```python
from build123d import *

# Parameters (mm, degrees)
BOSS_EXTRUDE1_DEPTH = 9
FILLET1_R           = 6
FILLET2_R           = 4
BOSS_EXTRUDE2_DEPTH = 18
LPATTERN1_COUNT     = 6
LPATTERN1_PITCH     = 6
CUT_EXTRUDE1_DEPTH  = 149.120803233
CUT_EXTRUDE2_DEPTH  = 8
SKETCH6_R           = 1.5
CUT_EXTRUDE3_DEPTH  = 149.120803233
SKETCH7_R           = 1.75
BOSS_EXTRUDE3_DEPTH = 3
SKETCH9_R           = 1.25
CUT_EXTRUDE4_DEPTH  = 1
SKETCH10_R          = 1.25
CUT_EXTRUDE5_DEPTH  = 1
CUT_EXTRUDE7_DEPTH  = 1


with BuildPart() as part:
    # Sketch2 → Boss-Extrude1 (new, symmetric)
    with BuildSketch(Plane(origin=(0, 0, 0), x_dir=(1, 0, 0), z_dir=(0, 1, 0))):
        with BuildLine():
            Line((-39.563995826, -83.832935468), (-42.630019208, -84.799815256))
            Line((-42.630019208, -84.799815256), (-45.240501853, -94.451735935))
            Line((-45.240501853, -94.451735935), (-34.884360154, -102.309873698))
            Line((-34.884360154, -102.309873698), (-25.888982114, -130.929502869))
            Line((-25.888982114, -130.929502869), (-25.888982114, -137.929502869))
            Line((-25.888982114, -137.929502869), (-14.888982114, -137.929502869))
            Line((-14.888982114, -137.929502869), (-14.888982114, -87.929502869))
            Line((-14.888982114, -87.929502869), (-6.735604792, -82.139646373))
            ThreePointArc((-6.735604792, -82.139646373), (-0.446003435, -73.378982845), (-11.226689216, -73.670744316))
            Line((-11.226689216, -73.670744316), (-21.363708344, -80.271037279))
            Line((-21.363708344, -80.271037279), (-28.269041415, -80.271037279))
            Line((-28.269041415, -80.271037279), (-28.269041415, -9.271037279))
            Line((-28.269041415, -9.271037279), (-51.831492155, -13.832935468))
            Line((-51.831492155, -13.832935468), (-39.563995826, -83.832935468))
        make_face()
    extrude(amount=BOSS_EXTRUDE1_DEPTH, both=True)

    # Fillet1
    fillet1_edges = [part.edges().sort_by_distance(p)[0] for p in [
        (-51.831492155, 0, 13.832935468),
        (-28.269041415, 0, 9.271037279),
    ]]
    fillet(fillet1_edges, radius=FILLET1_R)

    # Fillet2
    fillet2_edges = [part.edges().sort_by_distance(p)[0] for p in [
        (-42.630019208, 0, 84.799815256),
        (-25.888982114, 0, 137.929502869),
        (-45.240501853, 0, 94.451735935),
    ]]
    fillet(fillet2_edges, radius=FILLET2_R)

    # Sketch3 → Boss-Extrude2 (add)
    with BuildSketch(Plane(origin=(0, 9, 0), x_dir=(1, 0, 0), z_dir=(0, 1, 0))):
        Polygon((-14.888982114, -130.986597937), (-14.888982114, -134.986597937), (-10.884332588, -132.931354664), align=None)
    boss_extrude2 = extrude(amount=-BOSS_EXTRUDE2_DEPTH)

    # LPattern1: Boss-Extrude2 ×6
    with Locations(*[(0, 0, -i * LPATTERN1_PITCH) for i in range(1, LPATTERN1_COUNT)]):
        add(boss_extrude2)

    # Sketch4 → Cut-Extrude1 (cut, through all)
    with BuildSketch(Plane(origin=(0, 9, 0), x_dir=(1, 0, 0), z_dir=(0, 1, 0))):
        Polygon((-16.683079676, -131.183487283), (-16.683079676, -106.183487283), (-31.683079676, -106.183487283), align=None)
    extrude(amount=-CUT_EXTRUDE1_DEPTH, mode=Mode.SUBTRACT)

    # Sketch5 → Cut-Extrude2 (cut)
    with BuildSketch(Plane(origin=(-61.013660914, 0, 19.177080956), x_dir=(0.29984593468383275, 0, 0.9539876390465334), z_dir=(-0.9539876390465333, 0, 0.2998459346838327))):
        Polygon((94.142421284, 6), (94.142421284, -6), (112.142421284, -7.790586592), (112.142421284, 6.177981397), align=None)
    extrude(amount=-CUT_EXTRUDE2_DEPTH, mode=Mode.SUBTRACT)

    # Sketch6 → Cut-Extrude3 (cut, through all)
    with BuildSketch(Plane(origin=(0, 9, 0), x_dir=(1, 0, 0), z_dir=(0, 1, 0))):
        with Locations(Location((-44.904072418, -18.603144546, 0), (0, 0, 270))):
            Circle(SKETCH6_R)
    extrude(amount=-CUT_EXTRUDE3_DEPTH, mode=Mode.SUBTRACT)

    # Sketch7 → Boss-Extrude3 (add)
    with BuildSketch(Plane(origin=(0, 9, 0), x_dir=(1, 0, 0), z_dir=(0, 1, 0))):
        with Locations(Location((-40.67557748, -92.894380322, 0), (0, 0, 90))):
            Circle(SKETCH7_R)
        with Locations(Location((-5.76397205, -76.199117717, 0), (0, 0, 90))):
            Circle(SKETCH7_R)
    boss_extrude3 = extrude(amount=BOSS_EXTRUDE3_DEPTH)

    # Sketch9 → Cut-Extrude4 (cut)
    with BuildSketch(Plane(origin=(0, 12, 0), x_dir=(1, 0, 0), z_dir=(0, 1, 0))):
        with Locations(Location((-40.67557748, -92.894380322, 0), (0, 0, 270))):
            Circle(SKETCH9_R)
    cut_extrude4 = extrude(amount=-CUT_EXTRUDE4_DEPTH, mode=Mode.SUBTRACT)

    # Sketch10 → Cut-Extrude5 (cut)
    with BuildSketch(Plane(origin=(0, 12, 0), x_dir=(1, 0, 0), z_dir=(0, 1, 0))):
        with Locations(Location((-5.76397205, -76.199117717, 0), (0, 0, 270))):
            Circle(SKETCH10_R)
    cut_extrude5 = extrude(amount=-CUT_EXTRUDE5_DEPTH, mode=Mode.SUBTRACT)

    # Sketch11 → Cut-Extrude7 (cut)
    with BuildSketch(Plane(origin=(0, 9, 0), x_dir=(1, 0, 0), z_dir=(0, 1, 0))):
        with BuildLine():
            Line((-38.170562816, -25.535404597), (-32.594288437, -76.059830025))
            ThreePointArc((-32.594288437, -76.059830025), (-34.244390745, -78.119356213), (-36.303916933, -76.469253906))
            Line((-36.303916933, -76.469253906), (-41.880191311, -25.944828478))
            ThreePointArc((-41.880191311, -25.944828478), (-40.230089004, -23.88530229), (-38.170562816, -25.535404597))
        make_face()
    cut_extrude7 = extrude(amount=-CUT_EXTRUDE7_DEPTH, mode=Mode.SUBTRACT)

    # Mirror1: Boss-Extrude3, Cut-Extrude4, Cut-Extrude5, Cut-Extrude7 across plane
    add(boss_extrude3.mirror(Plane.ZX))
    add(cut_extrude4.mirror(Plane.ZX), mode=Mode.SUBTRACT)
    add(cut_extrude5.mirror(Plane.ZX), mode=Mode.SUBTRACT)
    add(cut_extrude7.mirror(Plane.ZX), mode=Mode.SUBTRACT)


solid = part.part
```
Verification items for the finished model (mm, model axes). A direction names the side the tool comes from. Give positions to 0.01 mm unless a question says otherwise; leave off trailing zeros. Loops run counter-clockwise (first coordinate to the right, second up) from the corner with the lowest first, then second, coordinate; pieces in that order, holes last. Notation, with made-up numbers: M -5,27.25 L 32,27.25 A14 cw 32,48.25 Z; hole C -1,67 d1. An arc over 180 degrees is marked long. One line per question, with ' | ' between items.
Item 1: Section check A-A, the plane z = 42.5. Record the cut outline in (x, y).
Completed:
outline: M -46.81,-9 L -40.05,-9 L -40.05,-8 L -36.3,-8 L -36.3,-9 L -28.27,-9 L -28.27,9 L -36.3,9 L -36.3,8 L -40.05,8 L -40.05,9 L -46.81,9 Z
Item 2: Section check B-B, the plane z = 63. Record the cut outline in (x, y).
Completed:
outline: M -43.21,-9 L -37.79,-9 L -37.79,-8 L -34.04,-8 L -34.04,-9 L -28.27,-9 L -28.27,9 L -34.04,9 L -34.04,8 L -37.79,8 L -37.79,9 L -43.21,9 Z
Item 3: Depth check by flat-ended pin: P1, Ø12, axis at y = 8, z = 116, coming from the -X side; P2, Ø3, axis at x = -5.76, z = 76.2, coming from the +Y side; P3, Ø2, axis at x = -37, z = 39, coming from the -Y side; P4, Ø3.5, axis at y = 4, z = 132, coming from the -X side. Enter the tip coordinate at first touch or a pass-through.
Completed:
P1: stops at x = -32.47 | P2: stops at y = 12 | P3: stops at y = -9 | P4: stops at x = -26.1
Item 4: Tool access check on faces 1 (the face through (-37, 8, 51)), 2 (the face through (-12.86, 0.13, 113.97)), 3 (the face through (-16.683, 0, 119)), 4 (the face through (-14.889, 0, 136)), 5 (the face through (-39.622, -11.507, 93.566)). Record the directions out of +Z, -Z, +X, -X, +Y, -Y that give a thin tool (end or side, any length) a straight path to the whole face; none if there is none.
Completed:
face 1: +Y | face 2: +X, +Y, -Y | face 3: +Y, -Y | face 4: +Z, +X, +Y, -Y | face 5: -Y
Item 5: Thickness scan on line 1 (Y direction, x = -29, z = 80.5); line 2 (X direction, y = -6, z = 115); line 3 (Z direction, x = -28, y = -4). Record the ranges inside material, lowest first. Write a range as [from, to].
Completed:
line 1: y = [-9, 9] | line 2: x = [-16.68, -11.02] | line 3: z = [80.27, 106.18]
Item 6: Draft check along X on faces 6 (the face through (-6, 11, 76)), 7 (the face through (-12.91, 0.13, 109.97)), 8 (the face through (-40.65, 0.13, 11.67)). Enter one of: +X half, -X half, draft (parallel to the pull), parting line (faces both ways), or undercut.
Completed:
face 6: undercut | face 7: +X half | face 8: -X half
